Design review of the part built by this model. Coordinates are the model's own, in mm. A direction names the side the tool comes from. Give positions to 0.01 mm unless a question says otherwise; leave off trailing zeros. Write each loop counter-clockwise with the first axis right and the second up, starting at its lowest first coordinate (ties: lowest second). Pieces come first, ordered by that corner, then holes. Notation, with made-up numbers: (61, 87) -> (82, 87) arc R23 ccw to (82, 99) -> close; hole circle Ø5 at (37.5, 30). An arc over 180 degrees is marked (long way). Return JSON: item names as keys, results as strings. Group by question number.
from build123d import *

# Parameters (mm, degrees)
SALIENTE_EXTRUIR1_DEPTH   = 15
SALIENTE_EXTRUIR1_2_DEPTH = 15
SALIENTE_EXTRUIR1_3_DEPTH = 15
SALIENTE_EXTRUIR1_4_DEPTH = 15
CORTAR_EXTRUIR1_REACH     = 68.288
CROQUIS3_W                = 25
CROQUIS3_H                = 10


with BuildPart() as part:
    # Croquis1 → Saliente-Extruir1 (new body)
    with BuildSketch(Plane.XY):
        with BuildLine():
            Line((-4.324392398, 38.256367187), (-4.492875219, 39.746875))
            ThreePointArc((-4.492875219, 39.746875), (-29.830479453, 26.648498937), (-40, 0))
            Line((-40, 0), (-38.5, 0))
            ThreePointArc((-38.5, 0), (-28.711836473, 25.649180227), (-4.324392398, 38.256367187))
        make_face()
    extrude(amount=SALIENTE_EXTRUIR1_DEPTH)



with BuildPart() as body_2:
    # Croquis1 → Saliente-Extruir1 2 (new body)
    with BuildSketch(Plane.XY):
        with BuildLine():
            Line((-38.256367187, -4.324392398), (-39.746875, -4.492875219))
            ThreePointArc((-39.746875, -4.492875219), (-26.648498937, -29.830479453), (0, -40))
            Line((0, -40), (0, -38.5))
            ThreePointArc((0, -38.5), (-25.649180227, -28.711836473), (-38.256367187, -4.324392398))
        make_face()
    extrude(amount=SALIENTE_EXTRUIR1_2_DEPTH)


with BuildPart() as body_3:
    # Croquis1 → Saliente-Extruir1 3 (new body)
    with BuildSketch(Plane.XY):
        with BuildLine():
            ThreePointArc((39.746875, 4.492875219), (26.648498937, 29.830479453), (0, 40))
            Line((0, 40), (0, 38.5))
            ThreePointArc((0, 38.5), (25.649180227, 28.711836473), (38.256367187, 4.324392398))
            Line((38.256367188, 4.324392398), (39.746875, 4.492875219))
        make_face()
    extrude(amount=SALIENTE_EXTRUIR1_3_DEPTH)


with BuildPart() as body_4:
    # Croquis1 → Saliente-Extruir1 4 (new body)
    with BuildSketch(Plane.XY):
        with BuildLine():
            ThreePointArc((4.492875219, -39.746875), (29.830479453, -26.648498937), (40, 0))
            Line((40, 0), (38.5, 0))
            ThreePointArc((38.5, 0), (28.711836473, -25.649180227), (4.324392398, -38.256367188))
            Line((4.324392398, -38.256367188), (4.492875219, -39.746875))
        make_face()
    extrude(amount=SALIENTE_EXTRUIR1_4_DEPTH)


with BuildPart() as part_1:
    add(part.part)

    add(body_2.part)  # Revoluci_n1 merges body 2

    add(body_3.part)  # Revoluci_n1 merges body 3

    add(body_4.part)  # Revoluci_n1 merges body 4
    # Croquis2 → Revoluci_n1 (revolve)
    with BuildSketch(Plane(origin=(0, 0, 0), x_dir=(1, 0, 0), z_dir=(0, 1, 0)), mode=Mode.PRIVATE) as revoluci_n1_sk:
        Polygon((-40, 0), (-45.656854249, 5.656854249), (-43.535533906, 7.778174593), (-35.757359313, 0), align=None)
    revolve(revoluci_n1_sk.sketch.rotate(Axis((0, 0, 0), (0, 0, -1)), 180), axis=Axis((0, 0, 0), (0, 0, -1)))

    # Croquis3 → Cortar-Extruir1 (cut, up to next)
    with BuildSketch(Plane(origin=(0, 0, 0), x_dir=(1, 0, 0), z_dir=(0, 1, 0)), mode=Mode.PRIVATE) as cortar_extruir1_sk1:
        with Locations((8.5, -8)):
            Rectangle(CROQUIS3_W, CROQUIS3_H)
    cortar_extruir1_tool1 = extrude(cortar_extruir1_sk1.sketch, amount=-CORTAR_EXTRUIR1_REACH, mode=Mode.PRIVATE) & part_1.part
    add(cortar_extruir1_tool1.solids().sort_by_distance((8.5, 0, 8))[0], mode=Mode.SUBTRACT)


solid = part_1.part
Q1. For L1, parallel to Y at x = -25, z = -5; L2, parallel to Y at x = 5, z = 13.25; L3, parallel to X at y = 21.5, z = 8, list the stretches that pass through material, from the lowest coordinate up. Write a range as from..to.
Q2. Tool access review of faces 5 (the face through (-29.56, 26.95, 7.4)), 6 (the face through (-25.355, -28.972, 7.395)), 7 (the face through (33.52, -21.83, 7.4)), 8 (the face through (26.95, 29.56, 7.4)): name each direction out of +Z, -Z, +X, -X, +Y, -Y from which nothing blocks a thin tool from reaching the whole face with its end or side.
Q3. Take a section at B-B, the plane z = -2. Give the boundary of the cut face in (x, y), plus the area to 3 significant figures.
Q4. Insertion check: pin 1 (1 mm diameter, centred on x = -32, y = 15, fed in from -Z); pin 2 (6 mm diameter, centred on y = -19.5, z = -3.5, fed in from -X); pin 3 (5 mm diameter, centred on y = 27.5, z = -1.5, fed in from -X). Each pin has a flat end and moves straight along its axis. Give the tip position at first contact, or say it passes through.
Q5. Take a section at A-A, the plane z = 7.25. Give the boundary of the cut face in (x, y), plus the area to 3 significant figures.
Q6. Mouldability with a two-part tool opening along X and no side actions: class faces 1 (the face through (38.49, -12.121, -0.354)), 2 (the face through (32.68, -20.35, 7.4)), 3 (the face through (-26, -29, 15)), 4 (the face through (25.355, 28.972, 7.395)) as +X half, -X half, draft (parallel to the pull), parting line (faces both ways), or undercut.
Final values:
{
 "1": {"L1": "y = -37.42..-32.19, 32.19..37.42", "L2": "y = -39.69..-38.17, 38.17..39.69", "L3": "x = -33.73..-31.94, 31.94..33.73"},
 "2": {"face 5": "+Z, -X, +Y", "face 6": "+Z", "face 7": "+Z, +X, -Y", "face 8": "+Z, +X, +Y"},
 "3": {"outline": "circle Ø84 at (0, 0); hole circle Ø75.51 at (0, 0)", "area": "1,060 mm²"},
 "4": {"pin 1": "stops at z = -0.08", "pin 2": "stops at x = -42.21", "pin 3": "stops at x = -34.89"},
 "5": {"outline": "(-40, 0) -> (-38.5, 0) arc R38.5 cw to (-4.32, 38.26) -> (-4.49, 39.75) arc R40 ccw to start; (-39.75, -4.49) arc R40 ccw to (0, -40) -> (0, -38.5) arc R38.5 cw to (-38.26, -4.32) -> close; (0, 38.5) arc R38.5 cw to (38.26, 4.32) -> (39.75, 4.49) arc R40 ccw to (0, 40) -> close; (21, -34.04) arc R40 ccw to (40, 0) -> (38.5, 0) arc R38.5 cw to (21, -32.27) -> close", "area": "317 mm²"},
 "6": {"face 1": "parting line", "face 2": "undercut", "face 3": "draft", "face 4": "undercut"}
}
